The model under review builds one solid part; all positions refer to its coordinate system, in mm. Face numbers are marked on the shaded views. Give positions to 0.01 mm unless a question says otherwise; leave off trailing zeros. Order: outer loops, then holes, each group sorted by start corner. A loop starts at its lowest first (then second) coordinate and runs counter-clockwise, first axis right, second up. Notation, with made-up numbers: (71, 10.25) - (115, 10.25) arc R25 cw to (115, 45.25) - close; hole circle Ø10 at (85.5, 86.5). An arc over 180 degrees is marked (long way). Use CSV: the item, a comma, the result in double quotes. Start each with the question number.
1. Take a section at B-B, the plane z = -6. State the section outline as (x, y) points, then the cut area to 3 significant figures.
2. For pin 1 (1.5 mm diameter, centred on y = 1.5, z = -14.5, fed in from +X); pin 2 (1.5 mm diameter, centred on y = 3, z = 11, fed in from -X); pin 3 (2.5 mm diameter, centred on y = 1.5, z = 12.5, fed in from +X), all flat-tipped, find the tip position at first contact; note any pin that passes through.
3. Draft analysis for pull direction X (two halves, no side actions). For the marked faces 1, 2 and 3, state which applies: released by +X, released by -X, zero draft, split by the parting line, or undercut.
4. To check wall thickness, follow line 1 (Z direction, x = 16.5, y = 1.8); line 2 (Z direction, x = -24.5, y = 2.3); line 3 (X direction, y = 2.2, z = -5). State the ranges of each line that lie inside material, in increasing order. Write a range as [from, to].
5. Take a section at C-C, the plane x = -33. State the section outline as (y, z) points, then the cut area to 3 significant figures.
6. Take a section at D-D, the plane x = -10. State the section outline as (y, z) points, then the cut area to 3 significant figures.
7. Take a section at A-A, the plane x = 15. State the section outline as (y, z) points, then the cut area to 3 significant figures.
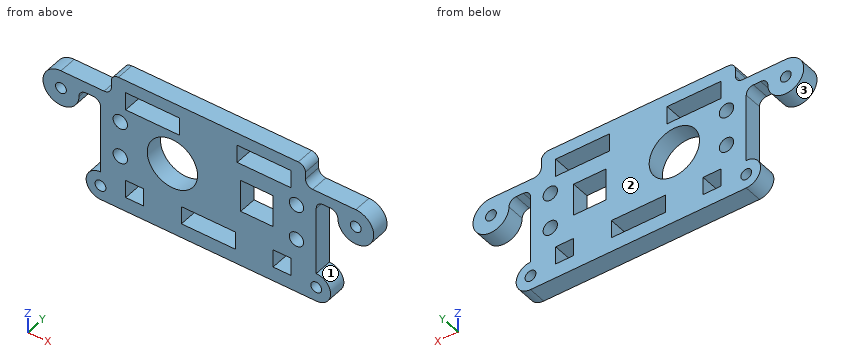
```python
from build123d import *

# Parameters (mm, degrees)
SKETCH1_R           = 7
SKETCH1_R_2         = 1.5
SKETCH1_R_3         = 2
SKETCH1_W           = 5
SKETCH1_H           = 5
SKETCH1_W_2         = 15
SKETCH1_W_3         = 9
SKETCH1_H_2         = 9
BOSS_EXTRUDE1_DEPTH = 5


with BuildPart() as part:
    # Sketch1 → Boss-Extrude1 (new body)
    with BuildSketch(Plane(origin=(0, 0, 0), x_dir=(1, 0, 0), z_dir=(0, 1, 0))):
        with BuildLine():
            Line((-29, -11.75), (-30, -11.75))
            Line((-30, -11.75), (-41, -11.75))
            ThreePointArc((-41, -11.75), (-44.535533906, -3.214466094), (-36, -6.75))
            ThreePointArc((-36, -6.75), (-35.414213562, -8.164213562), (-34, -8.75))
            Line((-34, -8.75), (-32, -8.75))
            ThreePointArc((-32, -8.75), (-30.585786438, -8.164213562), (-30, -6.75))
            Line((-30, -6.75), (-30, 12.25))
            ThreePointArc((-30, 12.25), (-34, 16.25), (-30, 20.25))
            Line((-30, 20.25), (30, 20.25))
            ThreePointArc((30, 20.25), (34, 16.25), (30, 12.25))
            Line((30, 12.25), (30, -6.75))
            ThreePointArc((30, -6.75), (30.585786438, -8.164213562), (32, -8.75))
            Line((32, -8.75), (34, -8.75))
            ThreePointArc((34, -8.75), (35.414213562, -8.164213562), (36, -6.75))
            ThreePointArc((36, -6.75), (44.535533906, -3.214466094), (41, -11.75))
            Line((41, -11.75), (30, -11.75))
            Line((30, -11.75), (29, -11.75))
            ThreePointArc((29, -11.75), (27.585786438, -12.335786438), (27, -13.75))
            Line((27, -13.75), (27, -15.75))
            ThreePointArc((27, -15.75), (26.414213562, -17.164213562), (25, -17.75))
            Line((25, -17.75), (-25, -17.75))
            ThreePointArc((-25, -17.75), (-26.414213562, -17.164213562), (-27, -15.75))
            Line((-27, -15.75), (-27, -13.75))
            ThreePointArc((-27, -13.75), (-27.585786438, -12.335786438), (-29, -11.75))
        make_face()
        with Locations((-10, 0)):
            Circle(SKETCH1_R, mode=Mode.SUBTRACT)
        with Locations((-30, 16.25)):
            Circle(SKETCH1_R_2, mode=Mode.SUBTRACT)
        with Locations((30, 16.25)):
            Circle(SKETCH1_R_2, mode=Mode.SUBTRACT)
        with Locations((41, -6.75)):
            Circle(SKETCH1_R_2, mode=Mode.SUBTRACT)
        with Locations((-41, -6.75)):
            Circle(SKETCH1_R_2, mode=Mode.SUBTRACT)
        with Locations((-24.5, -5)):
            Circle(SKETCH1_R_3, mode=Mode.SUBTRACT)
        with Locations((24.5, -5)):
            Circle(SKETCH1_R_3, mode=Mode.SUBTRACT)
        with Locations((-24.5, 5)):
            Circle(SKETCH1_R_3, mode=Mode.SUBTRACT)
        with Locations((24.5, 5)):
            Circle(SKETCH1_R_3, mode=Mode.SUBTRACT)
        with Locations((-20.5, 13.75)):
            Rectangle(SKETCH1_W, SKETCH1_H, mode=Mode.SUBTRACT)
        with Locations((0, 13.75)):
            Rectangle(SKETCH1_W_2, SKETCH1_H, mode=Mode.SUBTRACT)
        with Locations((20.5, 13.75)):
            Rectangle(SKETCH1_W, SKETCH1_H, mode=Mode.SUBTRACT)
        with Locations((-15.5, -11.75)):
            Rectangle(SKETCH1_W_2, SKETCH1_H, mode=Mode.SUBTRACT)
        with Locations((15.5, -11.75)):
            Rectangle(SKETCH1_W_2, SKETCH1_H, mode=Mode.SUBTRACT)
        with Locations((13.5, 0)):
            Rectangle(SKETCH1_W_3, SKETCH1_H_2, mode=Mode.SUBTRACT)
    extrude(amount=BOSS_EXTRUDE1_DEPTH)


solid = part.part
```
Determined:
1,outline,"(-30, 0) - (-26.23, 0) - (-26.23, 5) - (-30, 5) - close; (-22.77, 0) - (-13.61, 0) - (-13.61, 5) - (-22.77, 5) - close; (-6.39, 0) - (22.77, 0) - (22.77, 5) - (-6.39, 5) - close; (26.23, 0) - (30, 0) - (30, 5) - (26.23, 5) - close"
1,area,"229 mm²"
2,pin 1,"stops at x = 33.87"
2,pin 2,"stops at x = -44.57"
2,pin 3,"stops at x = 43.18"
3,face 1,"released by +X"
3,face 2,"zero draft"
3,face 3,"undercut"
4,line 1,"z = [-20.25, -4.5], [4.5, 9.25], [14.25, 17.75]"
4,line 2,"z = [-20.25, -7], [-3, 3], [7, 17.75]"
4,line 3,"x = [-30, -26.5], [-22.5, -14.9], [-5.1, 22.5], [26.5, 30]"
5,outline,"(0, -18.9) - (5, -18.9) - (5, -13.6) - (0, -13.6) - close; (0, 8.75) - (5, 8.75) - (5, 11.75) - (0, 11.75) - close"
5,area,"41.5 mm²"
6,outline,"(0, -20.25) - (5, -20.25) - (5, -7) - (0, -7) - close; (0, 7) - (5, 7) - (5, 9.25) - (0, 9.25) - close; (0, 14.25) - (5, 14.25) - (5, 17.75) - (0, 17.75) - close"
6,area,"95.0 mm²"
7,outline,"(0, -20.25) - (5, -20.25) - (5, -4.5) - (0, -4.5) - close; (0, 4.5) - (5, 4.5) - (5, 9.25) - (0, 9.25) - close; (0, 14.25) - (5, 14.25) - (5, 17.75) - (0, 17.75) - close"
7,area,"120 mm²"
